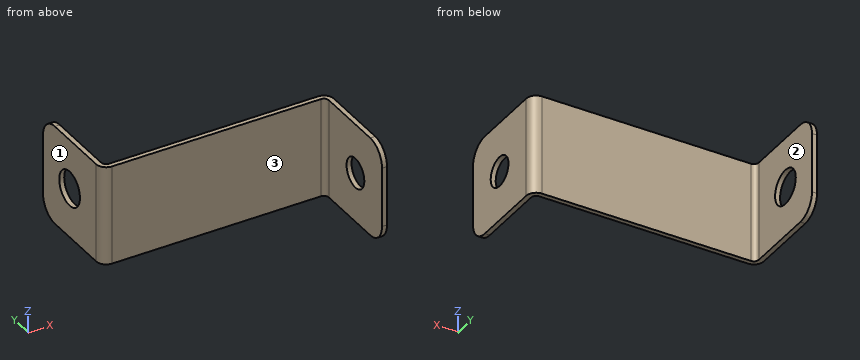
from build123d import *

# Parameters (mm, degrees)
SKETCH_1_W                       = 23
SKETCH_1_H                       = 10
EXTRUDE_1_DEPTH                  = 0.5
SM_EDGE_FLANGE_1_STRIP_W         = 3
SM_EDGE_FLANGE_1_STRIP_H         = 0.5
SM_EDGE_FLANGE_1_STRIP_CUT_DEPTH = 10
SM_EDGE_FLANGE_1_DEPTH           = 10
SM_EDGE_FLANGE_2_STRIP_W         = 3
SM_EDGE_FLANGE_2_STRIP_H         = 0.5
SM_EDGE_FLANGE_2_STRIP_CUT_DEPTH = 10
SM_EDGE_FLANGE_2_DEPTH           = 10
SKETCH_12_R                      = 1.5
CUT_EXTRUDE_1_DEPTH              = 0.5
SKETCH_13_R                      = 1.75
CUT_EXTRUDE_2_DEPTH              = 0.5
FILLET_1_R                       = 2


# Sheet-metal steps are written as plain solids
with BuildPart() as part:
    # Sketch 1 → Бобышка-Вытянуть1 (new body)
    with BuildSketch(Plane(origin=(0, 0, 0), x_dir=(1, 0, 0), z_dir=(0, 1, 0))):
        with Locations((-10.5, 0)):
            Rectangle(SKETCH_1_W, SKETCH_1_H)
    extrude(amount=EXTRUDE_1_DEPTH)

    # Ребро-кромка1 strip (across the edge) → Ребро-кромка1 strip cut (cut)
    with BuildSketch(Plane(origin=(1, 0, -5), x_dir=(-1, 0, 0), z_dir=(0, 0, 1))):
        with Locations((-0.5, -0.25)):
            Rectangle(SM_EDGE_FLANGE_1_STRIP_W, SM_EDGE_FLANGE_1_STRIP_H)
    extrude(amount=SM_EDGE_FLANGE_1_STRIP_CUT_DEPTH, mode=Mode.SUBTRACT)

    # Ребро-кромка1 section (across the edge) → Ребро-кромка1 (add)
    with BuildSketch(Plane(origin=(1, 0, -5), x_dir=(-1, 0, 0), z_dir=(0, 0, 1))):
        with BuildLine():
            Line((0, 0.5), (0, 9.5))
            Line((0, 9.5), (0.5, 9.5))
            Line((0.5, 9.5), (0.5, 0.5))
            ThreePointArc((0.5, 0.5), (0.646446609, 0.146446609), (1, 0))
            Line((1, 0), (1, -0.5))
            ThreePointArc((1, -0.5), (0.292893219, -0.207106781), (0, 0.5))
        make_face()
    extrude(amount=SM_EDGE_FLANGE_1_DEPTH)

    # Ребро-кромка2 strip (across the edge) → Ребро-кромка2 strip cut (cut)
    with BuildSketch(Plane(origin=(-22, 0.5, -5), x_dir=(1, 0, 0), z_dir=(0, 0, 1))):
        with Locations((-0.5, -0.25)):
            Rectangle(SM_EDGE_FLANGE_2_STRIP_W, SM_EDGE_FLANGE_2_STRIP_H)
    extrude(amount=SM_EDGE_FLANGE_2_STRIP_CUT_DEPTH, mode=Mode.SUBTRACT)

    # Ребро-кромка2 section (across the edge) → Ребро-кромка2 (add)
    with BuildSketch(Plane(origin=(-22, 0.5, -5), x_dir=(1, 0, 0), z_dir=(0, 0, 1))):
        with BuildLine():
            Line((0, 0.5), (0, 9.5))
            Line((0, 9.5), (0.5, 9.5))
            Line((0.5, 9.5), (0.5, 0.5))
            ThreePointArc((0.5, 0.5), (0.646446609, 0.146446609), (1, 0))
            Line((1, 0), (1, -0.5))
            ThreePointArc((1, -0.5), (0.292893219, -0.207106781), (0, 0.5))
        make_face()
    extrude(amount=SM_EDGE_FLANGE_2_DEPTH)

    # Эскиз12 → Вырез-Вытянуть1 (cut)
    with BuildSketch(Plane(origin=(1, 0, 0), x_dir=(0, 0, -1), z_dir=(1, 0, 0))):
        with Locations(Location((0, -5, 0), (0, 0, 90))):
            Circle(SKETCH_12_R)
    extrude(amount=-CUT_EXTRUDE_1_DEPTH, mode=Mode.SUBTRACT)

    # Эскиз13 → Вырез-Вытянуть2 (cut)
    with BuildSketch(Plane(origin=(-21.5, 0, 0), x_dir=(0, 0, -1), z_dir=(1, 0, 0))):
        with Locations(Location((0, 5.5, 0), (0, 0, 90))):
            Circle(SKETCH_13_R)
    extrude(amount=-CUT_EXTRUDE_2_DEPTH, mode=Mode.SUBTRACT)

    # Скругление1
    fillet_1_edges = [part.edges().sort_by_distance(p)[0] for p in [
        (0.75, -9.5, -5),
        (0.75, -9.5, 5),
        (-21.75, 10, -5),
        (-21.75, 10, 5),
    ]]
    fillet(fillet_1_edges, radius=FILLET_1_R)


solid = part.part
Here's how the part is built. I have some questions about the finished solid (model axes, mm). Face numbers are marked on the shaded views. A direction names the side the tool comes from. Coordinates: 2 decimals unless noted, no trailing zeros. Order: outer loops, then holes, each group sorted by start corner. A loop starts at its lowest first (then second) coordinate and runs counter-clockwise, first axis right, second up. Notation, with made-up numbers: (-22, -9) - (0, -9) arc R5 cw to (0, -1) - close; hole circle Ø10 at (-17.5, 39). An arc over 180 degrees is marked (long way). Use CSV: the item, a comma, the result in double quotes. Start each with the question number.
1. For the marked faces 1, 2 and 3, which set-ups out of +Z, -Z, +X, -X, +Y, -Y let a thin tool reach every point of the face, with its end or its side?
2. Suppose I cut it at C-C on y = 4.25. List the corners of the cut face in (x, z) for me, then the cut area to 3 significant figures.
3. Please list where these lines run through material, in increasing order: line 1 (Z direction, x = 0.9, y = -5); line 2 (Z direction, x = -21.8, y = 5.5); line 3 (Y direction, x = -5.5, z = 0). Write a range as from..to.
4. Suppose I cut it at D-D on y = -1.25. List the corners of the cut face in (x, z) for me, then the cut area to 3 significant figures.
5. I'm going to push flat-ended pins straight in: pin 1 (3 mm diameter, centred on x = -12, z = 1, fed in from +Y); pin 2 (2.5 mm diameter, centred on y = -4, z = 2, fed in from -X); pin 3 (1.5 mm diameter, centred on x = -4, z = 1.5, fed in from -Y); pin 4 (2 mm diameter, centred on y = 5.5, z = 0, fed in from -X). Where does each tip first touch, or does it pass through?
6. Suppose I cut it at A-A on y = -5. List the corners of the cut face in (x, z) for me, then the cut area to 3 significant figures.
7. Suppose I cut it at B-B on z = 0. List the corners of the cut face in (x, y) for me, then the cut area to 3 significant figures.
Output:
1,face 1,"+Z, -Z, -X, +Y, -Y"
1,face 2,"+Z, -Z, +X, +Y"
1,face 3,"+Z, -Z, -X, -Y"
2,outline,"(-22, -5) - (-21.5, -5) - (-21.5, -1.22) - (-22, -1.22) - close; (-22, 1.22) - (-21.5, 1.22) - (-21.5, 5) - (-22, 5) - close"
2,area,"3.78 mm2"
3,line 1,"z = -5..-1.5, 1.5..5"
3,line 2,"z = -5..-1.75, 1.75..5"
3,line 3,"y = 0..0.5"
4,outline,"(0.5, -5) - (1, -5) - (1, 5) - (0.5, 5) - close"
4,area,"5.00 mm2"
5,pin 1,"stops at y = 0.5"
5,pin 2,"stops at x = 0.5"
5,pin 3,"stops at y = 0"
5,pin 4,"passes through"
6,outline,"(0.5, -5) - (1, -5) - (1, -1.5) - (0.5, -1.5) - close; (0.5, 1.5) - (1, 1.5) - (1, 5) - (0.5, 5) - close"
6,area,"3.50 mm2"
7,outline,"(-22, 1) arc R1 ccw to (-21, 0) - (0, 0) arc R0.5 cw to (0.5, -0.5) - (0.5, -3.5) - (1, -3.5) - (1, -0.5) arc R1 ccw to (0, 0.5) - (-21, 0.5) arc R0.5 cw to (-21.5, 1) - (-21.5, 3.75) - (-22, 3.75) - close; (-22, 7.25) - (-21.5, 7.25) - (-21.5, 10) - (-22, 10) - close; (0.5, -9.5) - (1, -9.5) - (1, -6.5) - (0.5, -6.5) - close"
7,area,"17.4 mm2"
